```python
from build123d import *

# Parameters (mm, degrees)
F1_DEPTH = 44.45
F2_W     = 15.225
F2_H     = 63.5
F3_DEPTH = 7


with BuildPart() as f1:
    # F0 (on Right) → F1 (new body)
    with BuildSketch(Plane.YZ):
        Polygon((-25.589595, -3.175), (31.75, -3.175), (31.75, 3.175), (-31.75, 3.175), (-31.485815, -42.22507), (32.014185, -42.22507), (32.014185, -35.87507), (-25.589595, -35.433), align=None)
    extrude(amount=F1_DEPTH)

    # F2 (on face) → F3 (join)
    with BuildSketch(Plane(origin=(0, 0, -42.22507), x_dir=(1, 0, 0), z_dir=(0, 0, -1))):
        with Locations((36.8375, -0.264185)):
            Rectangle(F2_W, F2_H)
        with Locations((7.6125, -0.264185)):
            Rectangle(F2_W, F2_H)
    extrude(amount=F3_DEPTH)


solid = f1.part
```
CAD build for the part. Positions are in the model's coordinates, mm. A direction names the side the tool comes from. Coordinates: 2 decimals unless noted, no trailing zeros. Loops run counter-clockwise (first coordinate to the right, second up) from the corner with the lowest first, then second, coordinate; pieces in that order, holes last. Notation, with made-up numbers: (50.25, -19) - (84.25, -19) arc R17 ccw to (84.25, -12) - close; hole circle Ø3 at (-13.75, 89). An arc over 180 degrees is marked (long way). Use CSV: the item, a comma, the result in double quotes. Start each with the question number.
Q1. Two-plate mould, pull along X, no slides. Class faces 1 (the flat face through (22, 31.75, 0)), 2 (the flat face through (29.225, 1, -46)), 3 (the flat face through (0, -7, -40)): +X half, -X half, draft (parallel to the pull), parting line (faces both ways), or undercut.
Q2. 3-axis set-ups, long thin cutter, end or side, ignore diameter. For faces 4 (the flat face through (8, -31.486, -46)), 5 (the flat face through (22, 3, -3.175)), 6 (the flat face through (8, 0, -49.225)), 7 (the flat face through (15.225, 1, -46)), 8 (the flat face through (22, 0, 3.175)): which of +Z, -Z, +X, -X, +Y, -Y reach the whole face in a straight line?
Q3. Cut at A-A, the plane x = 33.5. List the corners of the cut face in (y, z) (3 decimals).
Q4. Cut at C-C, the plane y = 5. List the corners of the cut face in (x, z) (3 decimals).
Q5. Cut at B-B, the plane y = -16. List the corners of the cut face in (x, z) (3 decimals), then the cut area to 3 significant figures.
Q6. Cut at D-D, the plane z = -18.5. List the corners of the cut face in (x, y).
Q7. Probe probe 1 along X at (y, z) = (-20, -44) (3 decimals); probe 2 along Z at (x, y) = (3, -7) (3 decimals); probe 3 along Z at (x, y) = (39.5, 3.5) (3 decimals). List the from-to ranges inside material, lowest first. Write a range as from..to.
Q8. Drop flat-ended pins along their axis: P1, Ø1.5, axis at x = 32, z = -10.5, coming from the +Y side; P2, Ø3, axis at x = 20, z = -1.5, coming from the +Y side; P3, Ø5, axis at y = 18.5, z = -33, coming from the -X side; P4, Ø3.5, axis at x = 9.5, z = -47, coming from the -Y side. Give the stop position or say it passes through.
Here are the results:
1,face 1,"draft"
1,face 2,"undercut"
1,face 3,"-X half"
2,face 4,"-Z, +X, -X, -Y"
2,face 5,"+X, -X, +Y"
2,face 6,"-Z, +X, -X, +Y, -Y"
2,face 7,"-Z, +Y, -Y"
2,face 8,"+Z, +X, -X, +Y, -Y"
3,outline,"(-31.75, 3.175) - (-31.486, -42.225) - (-31.486, -49.225) - (32.014, -49.225) - (32.014, -35.875) - (-25.59, -35.433) - (-25.59, -3.175) - (31.75, -3.175) - (31.75, 3.175) - close"
4,outline,"(0, -49.225) - (15.225, -49.225) - (15.225, -42.225) - (29.225, -42.225) - (29.225, -49.225) - (44.45, -49.225) - (44.45, -35.668) - (0, -35.668) - close; (0, -3.175) - (44.45, -3.175) - (44.45, 3.175) - (0, 3.175) - close"
5,outline,"(0, -49.225) - (15.225, -49.225) - (15.225, -42.225) - (29.225, -42.225) - (29.225, -49.225) - (44.45, -49.225) - (44.45, -35.507) - (0, -35.507) - close; (0, -3.175) - (44.45, -3.175) - (44.45, 3.175) - (0, 3.175) - close"
5,area,"794 mm2"
6,outline,"(0, -31.62) - (44.45, -31.62) - (44.45, -25.59) - (0, -25.59) - close"
7,probe 1,"0..15.225, 29.225..44.45"
7,probe 2,"-49.225..-35.576, -3.175..3.175"
7,probe 3,"-49.225..-35.656, -3.175..3.175"
8,P1,"y = -25.59"
8,P2,"y = 31.75"
8,P3,"through"
8,P4,"y = -31.49"
